Could you check a few things on this drawing? It's one solid part, dimensions in mm from its lowest x, y, z. A direction names the side the tool comes from. Give positions to 0.01 mm unless a question says otherwise; leave off trailing zeros. Loops run counter-clockwise (first coordinate to the right, second up) from the corner with the lowest first, then second, coordinate; pieces in that order, holes last. Notation, with made-up numbers: M -30.75,70 L -1.75,70 A19 cw -1.75,103 Z; hole C -34.5,49.25 d5. An arc over 180 degrees is marked long. Return JSON: item names as keys, results as strings. Group by question number.
1. If we section it at C-C (z = 7.75): Write out the boundary of the cut face in (x, y) (1 decimal).
2. For pin 1 (3.5 mm diameter, centred on x = 14, z = 7, fed in from +Y); pin 2 (4 mm diameter, centred on x = 7, y = 11, fed in from +Z), each with a flat end and sliding along its axis, tell me the tip position at first contact or that it passes through.
3. If we section it at A-A (x = 10): Write out the boundary of the cut face in (y, z), plus the area to 3 significant figures.
4. Please list where these lines run through material, in increasing order: line 1 (Y direction, x = 10, z = 0.6); line 2 (Z direction, x = 18.25, y = 14.5).
5. If we section it at D-D (z = 1.75): Write out the boundary of the cut face in (x, y), plus the area to 3 significant figures.
6. If we mould it in two halves opening along Y, with no side actions, what happens to the marked faces 4, 5 and 6? For each: +Y half, -Y half, draft (parallel to the pull), parting line (faces both ways), or undercut.
7. If we section it at B-B (x = 14): Write out the boundary of the cut face in (y, z).
8. For the marked faces 1, 2 and 3, which set-ups out of +Z, -Z, +X, -X, +Y, -Y let a thin tool reach every point of the face, with its end or its side?
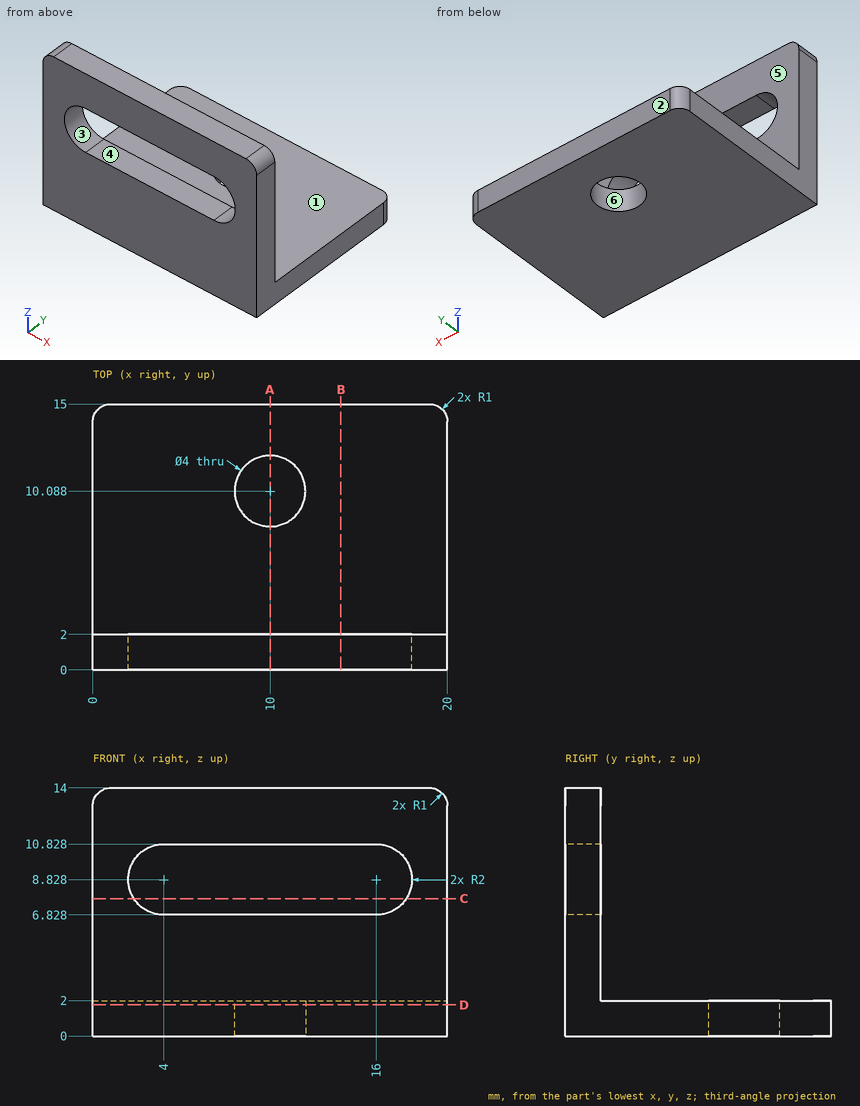
Answer:
{
 "1": {"outline": "M 0,0 L 2.3,0 L 2.3,2 L 0,2 Z; M 17.7,0 L 20,0 L 20,2 L 17.7,2 Z"},
 "2": {"pin 1": "stops at y = 2", "pin 2": "stops at z = 2"},
 "3": {"outline": "M 0,0 L 8.09,0 L 8.09,2 L 2,2 L 2,6.83 L 0,6.83 Z; M 0,10.83 L 2,10.83 L 2,14 L 0,14 Z; M 12.09,0 L 15,0 L 15,2 L 12.09,2 Z", "area": "38.0 mm²"},
 "4": {"line 1": "y = 0 to 8.09, 12.09 to 15", "line 2": "z = 0 to 2"},
 "5": {"outline": "M 0,0 L 20,0 L 20,14 A1 ccw 19,15 L 1,15 A1 ccw 0,14 Z; hole C 10,10.09 d4", "area": "287 mm²"},
 "6": {"face 4": "draft", "face 5": "+Y half", "face 6": "undercut"},
 "7": {"outline": "M 0,0 L 15,0 L 15,2 L 2,2 L 2,6.83 L 0,6.83 Z; M 0,10.83 L 2,10.83 L 2,14 L 0,14 Z"},
 "8": {"face 1": "+Z, +X, -X, +Y", "face 2": "+Z, -Z, +X, -X, +Y", "face 3": "+Y, -Y"}
}
